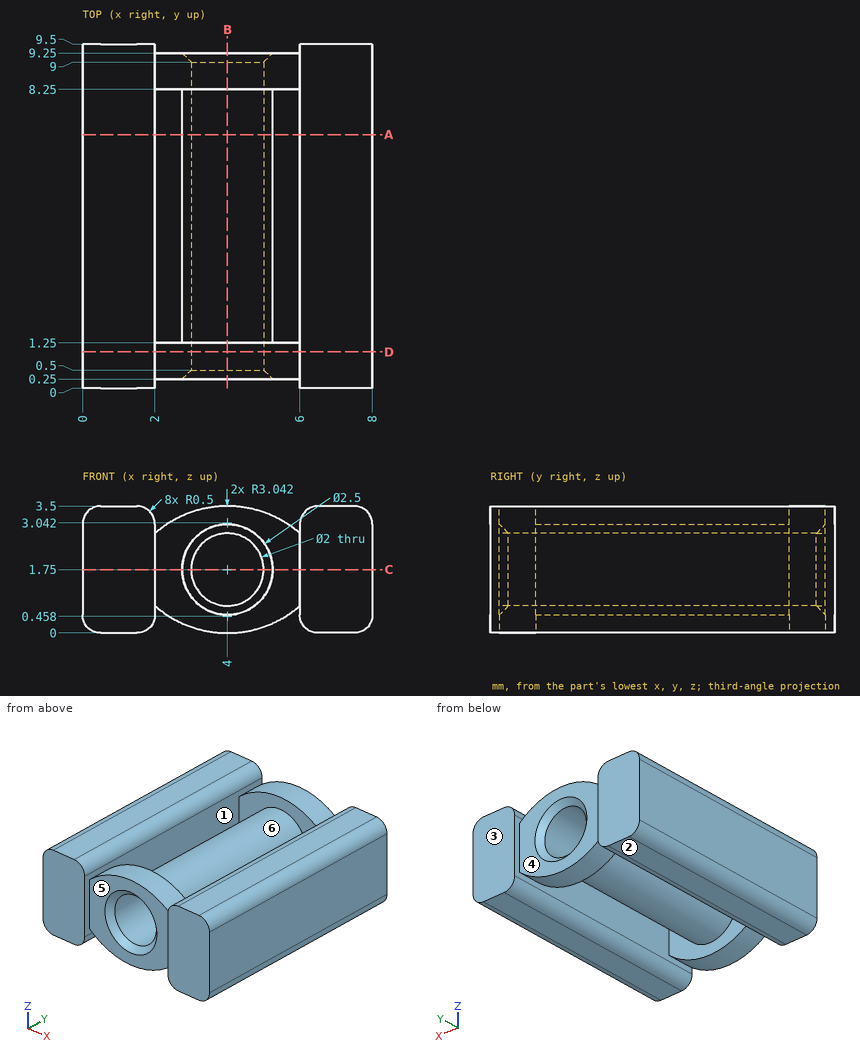
Answer from the drawing. Dimensions are ordinates in mm from the lowest x, y and z of the part. A direction names the side the tool comes from. Round coordinates to 2 decimals unless told otherwise and drop trailing zeros. Order: outer loops, then holes, each group sorted by start corner. A loop starts at its lowest first (then second) coordinate and runs counter-clockwise, first axis right, second up.
1) Straight lines are drawn through the part: L1, parallel to X at y = 3.25, z = 1.75; L2, parallel to Z at x = 4, y = 4.5; L3, parallel to X at y = 5, z = 0.85 (1 decimal). For each, find the intervals that lie inside material, in ascending order.
2) The part is cut by section B-B on x = 4. Write down the section's boundary in (y, z).
3) For the marked faces 4, 5 and 6, determine the directions among +Z, -Z, +X, -X, +Y, -Y from which every point of the face is accessible in a straight line to the end or side of a thin tool.
4) The part is cut by section A-A on y = 7. Write down the section's boundary in (x, z).
5) Flat-ended cylindrical pins translate along their axes: pin 1 (1 mm diameter, centred on x = 5, z = 2, fed in from +Y); pin 2 (1.7 mm diameter, centred on x = 3.5, z = 1, fed in from -Y). Find the tip coordinate at first contact, or state that the pin passes through.
6) The part is cut by section C-C on z = 1.75. Write down the section's boundary in (x, y).
7) The mould has two halves that part along Y. Classify the marked faces 1, 2 and 3: released by +Y, released by -Y, zero draft, split by the parting line, or undercut.
8) The part is cut by section D-D on y = 1. Write down the section's boundary in (x, z).
Resolved:
1. L1: x = 0 to 2, 2.75 to 3, 5 to 5.25, 6 to 8
1. L2: z = 0.5 to 0.75, 2.75 to 3
1. L3: x = 0 to 2, 3.1 to 3.6, 4.4 to 4.9, 6 to 8
2. outline: (0.25, 0) - (1.25, 0) - (1.25, 0.5) - (8.25, 0.5) - (8.25, 0) - (9.25, 0) - (9.25, 0.5) - (9, 0.75) - (0.5, 0.75) - (0.25, 0.5) - close; (0.25, 3) - (0.5, 2.75) - (9, 2.75) - (9.25, 3) - (9.25, 3.5) - (8.25, 3.5) - (8.25, 3) - (1.25, 3) - (1.25, 3.5) - (0.25, 3.5) - close
3. face 4: +Z, -Z, +Y
3. face 5: +Z, -Z, -Y
3. face 6: none
4. outline: (0, 0.5) arc R0.5 ccw to (0.5, 0) - (1.5, 0) arc R0.5 ccw to (2, 0.5) - (2, 3) arc R0.5 ccw to (1.5, 3.5) - (0.5, 3.5) arc R0.5 ccw to (0, 3) - close; circle Ø2.5 at (4, 1.75); (6, 0.5) arc R0.5 ccw to (6.5, 0) - (7.5, 0) arc R0.5 ccw to (8, 0.5) - (8, 3) arc R0.5 ccw to (7.5, 3.5) - (6.5, 3.5) arc R0.5 ccw to (6, 3) - close; hole circle Ø2 at (4, 1.75)
5. pin 1: stops at y = 9.25
5. pin 2: stops at y = 0.25
6. outline: (0, 0) - (2, 0) - (2, 0.25) - (2.75, 0.25) - (3, 0.5) - (3, 9) - (2.75, 9.25) - (2, 9.25) - (2, 9.5) - (0, 9.5) - close; (5, 0.5) - (5.25, 0.25) - (6, 0.25) - (6, 0) - (8, 0) - (8, 9.5) - (6, 9.5) - (6, 9.25) - (5.25, 9.25) - (5, 9) - close; hole (2, 1.25) - (2.75, 1.25) - (2.75, 8.25) - (2, 8.25) - close; hole (5.25, 1.25) - (6, 1.25) - (6, 8.25) - (5.25, 8.25) - close
7. face 1: undercut
7. face 2: zero draft
7. face 3: released by +Y
8. outline: (0, 0.5) arc R0.5 ccw to (0.5, 0) - (1.5, 0) arc R0.5 ccw to (2, 0.5) - (2, 0.75) arc R3.04 ccw to (6, 0.75) - (6, 0.5) arc R0.5 ccw to (6.5, 0) - (7.5, 0) arc R0.5 ccw to (8, 0.5) - (8, 3) arc R0.5 ccw to (7.5, 3.5) - (6.5, 3.5) arc R0.5 ccw to (6, 3) - (6, 2.75) arc R3.04 ccw to (2, 2.75) - (2, 3) arc R0.5 ccw to (1.5, 3.5) - (0.5, 3.5) arc R0.5 ccw to (0, 3) - close; hole circle Ø2 at (4, 1.75)
